```python
from build123d import *

# Parameters (mm, degrees)
SKETCH1_W              = 87
SKETCH1_H              = 80
PCB_DEPTH              = 2
SKETCH2_R              = 1.8
ATTACHMENT_HOLES_DEPTH = 3
LPATTERN1_COUNT        = 2
LPATTERN1_PITCH        = 70
LPATTERN1_COUNT_DIR2   = 2
LPATTERN1_PITCH_DIR2   = 70
SKETCH3_W              = 86.3
SKETCH3_H              = 53.3
IDUINO_DEPTH           = 10


with BuildPart() as part:
    # Sketch1 → PCB (new body)
    with BuildSketch(Plane(origin=(0, 0, 0), x_dir=(1, 0, 0), z_dir=(0, 1, 0))):
        with Locations((43.5, 40)):
            Rectangle(SKETCH1_W, SKETCH1_H)
    extrude(amount=PCB_DEPTH)

    # Sketch2 → Attachment Holes (cut, through all)
    with BuildSketch(Plane(origin=(0, 2, 0), x_dir=(1, 0, 0), z_dir=(0, 1, 0))):
        with Locations((9, 75)):
            Circle(SKETCH2_R)
    attachment_holes = extrude(amount=-ATTACHMENT_HOLES_DEPTH, mode=Mode.SUBTRACT)

    # LPattern1: Attachment Holes 2 × 2
    with Locations(*[(i * LPATTERN1_PITCH, 0, j * LPATTERN1_PITCH_DIR2) for i in range(LPATTERN1_COUNT) for j in range(LPATTERN1_COUNT_DIR2) if (i, j) != (0, 0)]):
        add(attachment_holes, mode=Mode.SUBTRACT)

    # Sketch3 → Iduino (add)
    with BuildSketch(Plane(origin=(0, 2, 0), x_dir=(1, 0, 0), z_dir=(0, 1, 0))):
        with Locations((43.65, 43.35)):
            Rectangle(SKETCH3_W, SKETCH3_H)
    extrude(amount=IDUINO_DEPTH)


solid = part.part
```
Model file for the job. Use its own axes, mm. A direction names the side the tool comes from. Coordinates: 2 decimals unless noted, no trailing zeros. Write each loop counter-clockwise with the first axis right and the second up, starting at its lowest first coordinate (ties: lowest second). Pieces come first, ordered by that corner, then holes. Notation, with made-up numbers: (48.25, 46.25) - (79.25, 46.25) arc R23 ccw to (79.25, 80.25) - close; hole circle Ø9 at (45, -18). An arc over 180 degrees is marked (long way). Use a Markdown table: item, result. Add a question column.
Item 1: Band-saw the part on B-B, the plane x = 79. Write the cut outline in (y, z).
Item 2: Two-plate mould, pull along X, no slides. Class faces 1 (the face through (9.968, 1.014, -76.518)), 2 (the face through (43, 2, -16)), 3 (the face through (0, 1, -39)): pulls with the +X half, pulls with the -X half, needs draft (parallel to the pull), parting line crosses it, or undercut.
Item 3: Drop flat-ended pins along their axis: pin 1 (6 mm diameter, centred on x = 79, z = -75, fed in from +Y); pin 2 (2 mm diameter, centred on y = 6.5, z = -30, fed in from -X); pin 3 (3 mm diameter, centred on y = 4.5, z = -58, fed in from +X). Give the stop position or say it passes through.
Item 4: 3-axis set-ups, long thin cutter, end or side, ignore diameter. For faces 4 (the face through (86.8, 7, -43)), 5 (the face through (43, 7, -16.7)), 6 (the face through (43, 7, -70)): which of +Z, -Z, +X, -X, +Y, -Y reach the whole face in a straight line?
Item 5: Band-saw the part on C-C, the plane y = 6.5. Write the cut outline in (x, z).
Item 6: Band-saw the part on A-A, the plane z = -5. Write the cut outline in (x, y).
Item 7: Drill centre lines: line 1 along Z through (x, y) = (79, 1.45); line 2 along X through (y, z) = (1.45, -5); line 3 along X through (y, z) = (4.25, -31.5). Where is each one in solid material? Low to high.
A:
| question | item | result |
|---|---|---|
| 1 | outline | (0, -80) - (2, -80) - (2, -76.8) - (0, -76.8) - close; (0, -73.2) - (2, -73.2) - (2, -70) - (12, -70) - (12, -16.7) - (2, -16.7) - (2, -6.8) - (0, -6.8) - close; (0, -3.2) - (2, -3.2) - (2, 0) - (0, 0) - close |
| 2 | face 1 | undercut |
| 2 | face 2 | needs draft |
| 2 | face 3 | pulls with the -X half |
| 3 | pin 1 | stops at y = 2 |
| 3 | pin 2 | stops at x = 0.5 |
| 3 | pin 3 | stops at x = 86.8 |
| 4 | face 4 | +Z, -Z, +X, +Y |
| 4 | face 5 | +Z, +X, -X, +Y |
| 4 | face 6 | -Z, +X, -X, +Y |
| 5 | outline | (0.5, -70) - (86.8, -70) - (86.8, -16.7) - (0.5, -16.7) - close |
| 6 | outline | (0, 0) - (7.2, 0) - (7.2, 2) - (0, 2) - close; (10.8, 0) - (77.2, 0) - (77.2, 2) - (10.8, 2) - close; (80.8, 0) - (87, 0) - (87, 2) - (80.8, 2) - close |
| 7 | line 1 | z = -80 to -76.8, -73.2 to -6.8, -3.2 to 0 |
| 7 | line 2 | x = 0 to 7.2, 10.8 to 77.2, 80.8 to 87 |
| 7 | line 3 | x = 0.5 to 86.8 |
